from build123d import *

# Parameters (mm, degrees)
SKETCH1_R           = 2
BOSS_EXTRUDE1_DEPTH = 1


with BuildPart() as part:
    # Sketch1 → Boss-Extrude1 (new body)
    with BuildSketch(Plane.XY):
        with BuildLine():
            Line((100.581340861, -63.068209116), (100.581340861, -13.788708514))
            ThreePointArc((100.581340861, -13.788708514), (99.995554423, -12.374494952), (98.581340861, -11.788708514))
            Line((98.581340861, -11.788708514), (6.526340861, -11.788708514))
            ThreePointArc((6.526340861, -11.788708514), (5.112127298, -12.374494952), (4.526340861, -13.788708514))
            Line((4.526340861, -13.788708514), (4.526340861, -63.063209116))
            ThreePointArc((4.526340861, -63.063209116), (4.374099926, -63.828575981), (3.940554423, -64.477422679))
            Line((3.940554423, -64.477422679), (-15.055177547, -83.473154649))
            ThreePointArc((-15.055177547, -83.473154649), (-15.48872305, -84.122001347), (-15.640963985, -84.887368211))
            Line((-15.640963985, -84.887368211), (-15.640963985, -104.958318205))
            ThreePointArc((-15.640963985, -104.958318205), (-15.055177547, -106.372531767), (-13.640963985, -106.958318205))
            Line((-13.640963985, -106.958318205), (118.743645706, -106.958318205))
            ThreePointArc((118.743645706, -106.958318205), (120.157859269, -106.372531767), (120.743645706, -104.958318205))
            Line((120.743645706, -104.958318205), (120.743645706, -84.887368211))
            ThreePointArc((120.743645706, -84.887368211), (120.591404771, -84.122001347), (120.157859269, -83.473154649))
            Line((120.157859269, -83.473154649), (101.167127298, -64.482422679))
            ThreePointArc((101.167127298, -64.482422679), (100.733581796, -63.833575981), (100.581340861, -63.068209116))
        make_face()
        with Locations((-12.195717461, -103.513071681)):
            Circle(SKETCH1_R, mode=Mode.SUBTRACT)
        with Locations((52.551340861, -103.658318205)):
            Circle(SKETCH1_R, mode=Mode.SUBTRACT)
        with Locations((117.297199097, -103.511871596)):
            Circle(SKETCH1_R, mode=Mode.SUBTRACT)
        with Locations((107.016568327, -74.998768464)):
            Circle(SKETCH1_R, mode=Mode.SUBTRACT)
        with Locations((-1.913886606, -74.998768464)):
            Circle(SKETCH1_R, mode=Mode.SUBTRACT)
        with Locations((7.97278747, -15.235155124)):
            Circle(SKETCH1_R, mode=Mode.SUBTRACT)
        with Locations((52.553840861, -15.088708514)):
            Circle(SKETCH1_R, mode=Mode.SUBTRACT)
        with Locations((97.134894251, -15.235155124)):
            Circle(SKETCH1_R, mode=Mode.SUBTRACT)
        with BuildLine():
            Line((98.781340861, -63.813793529), (98.781340861, -20.07225136))
            ThreePointArc((98.781340861, -20.07225136), (98.246194168, -18.710559476), (96.927136073, -18.0775725))
            ThreePointArc((96.927136073, -18.0775725), (95.119639925, -17.25040945), (94.292476875, -15.442913302))
            ThreePointArc((94.292476875, -15.442913302), (93.659489899, -14.123855207), (92.297798015, -13.588708514))
            Line((92.297798015, -13.588708514), (57.377998818, -13.588708514))
            ThreePointArc((57.377998818, -13.588708514), (56.03866524, -14.103385126), (55.388655331, -15.382522947))
            ThreePointArc((55.388655331, -15.382522947), (52.553840861, -17.938708514), (49.719026391, -15.382522947))
            ThreePointArc((49.719026391, -15.382522947), (49.069016481, -14.103385126), (47.729682903, -13.588708514))
            Line((47.729682903, -13.588708514), (12.809883707, -13.588708514))
            ThreePointArc((12.809883707, -13.588708514), (11.448191822, -14.123855207), (10.815204846, -15.442913302))
            ThreePointArc((10.815204846, -15.442913302), (9.988041797, -17.25040945), (8.180545648, -18.0775725))
            ThreePointArc((8.180545648, -18.0775725), (6.861487553, -18.710559476), (6.326340861, -20.07225136))
            Line((6.326340861, -20.07225136), (6.326340861, -63.808793529))
            ThreePointArc((6.326340861, -63.808793529), (6.174099926, -64.574160393), (5.740554423, -65.223007091))
            Line((5.740554423, -65.223007091), (0.436648028, -70.526913486))
            ThreePointArc((0.436648028, -70.526913486), (-0.146472505, -71.837896664), (0.298388107, -73.202010106))
            ThreePointArc((0.298388107, -73.202010106), (0.101367721, -77.01402279), (-3.710644963, -77.211043177))
            ThreePointArc((-3.710644963, -77.211043177), (-5.074758405, -76.766182564), (-6.385741583, -77.349303097))
            Line((-6.385741583, -77.349303097), (-13.255177547, -84.218739061))
            ThreePointArc((-13.255177547, -84.218739061), (-13.68872305, -84.867585759), (-13.840963985, -85.632952624))
            Line((-13.840963985, -85.632952624), (-13.840963985, -98.677765048))
            ThreePointArc((-13.840963985, -98.677765048), (-13.306003678, -100.039256399), (-11.987305288, -100.672403919))
            ThreePointArc((-11.987305288, -100.672403919), (-10.18166322, -101.49901744), (-9.355049698, -103.304659508))
            ThreePointArc((-9.355049698, -103.304659508), (-8.721902178, -104.623357898), (-7.360410828, -105.158318205))
            Line((-7.360410828, -105.158318205), (47.727182903, -105.158318205))
            ThreePointArc((47.727182903, -105.158318205), (49.066516481, -104.643641593), (49.716526391, -103.364503772))
            ThreePointArc((49.716526391, -103.364503772), (52.551340861, -100.808318205), (55.386155331, -103.364503772))
            ThreePointArc((55.386155331, -103.364503772), (56.03616524, -104.643641593), (57.375498818, -105.158318205))
            Line((57.375498818, -105.158318205), (112.46010286, -105.158318205))
            ThreePointArc((112.46010286, -105.158318205), (113.821794745, -104.623171513), (114.454781721, -103.304113418))
            ThreePointArc((114.454781721, -103.304113418), (115.28194477, -101.496617269), (117.089440919, -100.66945422))
            ThreePointArc((117.089440919, -100.66945422), (118.408499014, -100.036467243), (118.943645706, -98.674775359))
            Line((118.943645706, -98.674775359), (118.943645706, -85.632952624))
            ThreePointArc((118.943645706, -85.632952624), (118.791404771, -84.867585759), (118.357859269, -84.218739061))
            Line((118.357859269, -84.218739061), (111.488423304, -77.349303097))
            ThreePointArc((111.488423304, -77.349303097), (110.177440127, -76.766182564), (108.813326684, -77.211043177))
            ThreePointArc((108.813326684, -77.211043177), (105.001314001, -77.01402279), (104.804293614, -73.202010106))
            ThreePointArc((104.804293614, -73.202010106), (105.249154227, -71.837896664), (104.666033694, -70.526913486))
            Line((104.666033694, -70.526913486), (99.367127298, -65.228007091))
            ThreePointArc((99.367127298, -65.228007091), (98.933581796, -64.579160393), (98.781340861, -63.813793529))
        make_face(mode=Mode.SUBTRACT)
    extrude(amount=BOSS_EXTRUDE1_DEPTH)


solid = part.part
Input: part model. Units: mm. Frame: model coordinates. A direction names the side the tool comes from. Give positions to 0.01 mm unless a question says otherwise; leave off trailing zeros. Order: outer loops, then holes, each group sorted by start corner. A loop starts at its lowest first (then second) coordinate and runs counter-clockwise, first axis right, second up.
Q1. Ray query, probe 1 along X at (y, z) = (-92, 0.3); probe 2 along Y at (x, z) = (8, 0.75); probe 3 along X at (y, z) = (-37, 0.95). Return the intervals inside material, ascending.
Checked values:
probe 1: x = -15.64 to -13.84, 118.94 to 120.74
probe 2: y = -106.96 to -105.16, -18.1 to -17.23, -13.24 to -11.79
probe 3: x = 4.53 to 6.33, 98.78 to 100.58
Q2. Section C-C on z = 0.55. State how many separate pieces and enclosed holes the cut face has, and give its area (3 significant figures).
Checked values:
separate pieces: 1
enclosed holes: 9
area: 846 mm2
Q3. Draft query along Y for faces 3 (the flat face through (-5.42, -73.84, 0.49)), 4 (the flat face through (42, -13, 0)), 5 (the flat face through (102.05, -67.91, 0.49)). Return one class per face: +Y half, -Y half, draft (parallel to the pull), parting line (faces both ways), or undercut.
Checked values:
face 3: +Y half
face 4: draft
face 5: undercut
Q4. Section B-B on x = 40. Output: boundary loops of the cut face in (y, z), and give its area (3 significant figures).
Checked values:
outline: (-106.96, 0) - (-105.16, 0) - (-105.16, 1) - (-106.96, 1) - close; (-13.59, 0) - (-11.79, 0) - (-11.79, 1) - (-13.59, 1) - close
area: 3.60 mm2
Q5. Section A-A on y = -36.5. Output: boundary loops of the cut face in (x, z).
Checked values:
outline: (4.53, 0) - (6.33, 0) - (6.33, 1) - (4.53, 1) - close; (98.78, 0) - (100.58, 0) - (100.58, 1) - (98.78, 1) - close
Q6. Set-up query: faces 1 (the flat face through (110.795, -74.111, 0.493)), 2 (the cylindrical face through (-10.2, -101.48, 0.49)). Return all of +Z, -Z, +X, -X, +Y, -Y with unobstructed straight access to the full face (end or side cutting, diameter ignored); none if empty.
Checked values:
face 1: +Z, -Z, +X, +Y
face 2: +Z, -Z
Q7. Contact query for flat-ended pins moving along their axis: pin 1 Ø4.5 at (x, y) = (52.55, -103.66) entering from -Z; pin 2 Ø3 at (x, y) = (97.13, -15.24) entering from -Z. Output: stop coordinate, or through.
Checked values:
pin 1: stops at z = 0
pin 2: passes through
